from build123d import *

# Parameters (mm, degrees)
BOSS_EXTRUDE1_DEPTH = 2
EXTRUDE_1_DEPTH     = 5
EXTRUDE_2_DEPTH     = 5
SKETCH_4_R          = 14
SKETCH_4_R_2        = 14.00018903
CUT_EXTRUDE_1_DEPTH = 5
SKETCH1_3_R         = 10
CUT_EXTRUDE_2_DEPTH = 15
RIB_2_REACH         = 478.571
SKETCH_5_WALLS_W    = 5
SKETCH_5_WALLS_H    = 961.14191471
SKETCH_5_WALLS_H_2  = 961.14172568


with BuildPart() as part:
    # Sketch1 → Boss-Extrude1 (new, symmetric)
    with BuildSketch(Plane(origin=(0, 0, 0), x_dir=(0, 0, -1), z_dir=(1, 0, 0))):
        with BuildLine():
            Line((-48.878566689, 24.607830126), (451.121433311, 24.607830126))
            ThreePointArc((451.121433311, 24.607830126), (475.729263437, 0), (451.121433311, -24.607830126))
            Line((451.121433311, -24.607830126), (-48.878566689, -24.607830126))
            ThreePointArc((-48.878566689, -24.607830126), (-73.486396815, 0), (-48.878566689, 24.607830126))
        make_face()
    extrude(amount=BOSS_EXTRUDE1_DEPTH, both=True)

    # Sketch 1 → Extrude 1 (add)
    with BuildSketch(Plane(origin=(2, 0, 0), x_dir=(0, 0, -1), z_dir=(1, 0, 0))):
        with BuildLine():
            Line((451.121433311, 24.607830126), (-48.878566689, 24.607830126))
            ThreePointArc((-48.878566689, 24.607830126), (-73.486396815, 0), (-48.878566689, -24.607830126))
            Line((-48.878566689, -24.607830126), (451.121433311, -24.607830126))
            ThreePointArc((451.121433311, -24.607830126), (475.729263437, 0), (451.121433311, 24.607830126))
        make_face()
    extrude(amount=EXTRUDE_1_DEPTH)

    # Sketch 2 → Extrude 2 (add)
    with BuildSketch(Plane.ZY.offset(2)):
        with BuildLine():
            Line((-451.121433311, 24.607830126), (48.878566689, 24.607830126))
            ThreePointArc((48.878566689, 24.607830126), (73.486396815, 0), (48.878566689, -24.607830126))
            Line((48.878566689, -24.607830126), (-451.121433311, -24.607830126))
            ThreePointArc((-451.121433311, -24.607830126), (-475.729263437, 0), (-451.121433311, 24.607830126))
        make_face()
    extrude(amount=EXTRUDE_2_DEPTH)

    # Sketch 4 → Cut-Extrude 1 (cut)
    with BuildSketch(Plane.ZY.offset(7)):
        with BuildLine():
            ThreePointArc((48.878566689, 20), (68.878566689, 0), (48.878566689, -20))
            Line((48.878566689, -20), (-451.121433311, -20))
            ThreePointArc((-451.121433311, -20), (-471.121433311, 0), (-451.121433311, 20))
            Line((-451.121433311, 20), (48.878566689, 20))
        make_face()
        with Locations((48.878566689, 0)):
            Circle(SKETCH_4_R, mode=Mode.SUBTRACT)
        with Locations((-201.121433311, 0)):
            Circle(SKETCH_4_R_2, mode=Mode.SUBTRACT)
        with Locations((-451.121433311, 0)):
            Circle(SKETCH_4_R, mode=Mode.SUBTRACT)
    cut_extrude_1 = extrude(amount=-CUT_EXTRUDE_1_DEPTH, mode=Mode.SUBTRACT)

    # Mirror 1: Cut-Extrude 1 across plane
    add(cut_extrude_1.mirror(Plane.ZY), mode=Mode.SUBTRACT)

    # Sketch1_3 → Cut-Extrude 2 (cut, symmetric)
    with BuildSketch(Plane(origin=(0, 0, 0), x_dir=(0, 0, -1), z_dir=(1, 0, 0))):
        with Locations((-48.878566689, 0)):
            Circle(SKETCH1_3_R)
        with Locations((451.121433311, 0)):
            Circle(SKETCH1_3_R)
        with Locations((201.121433311, 0)):
            Circle(SKETCH1_3_R)
    extrude(amount=CUT_EXTRUDE_2_DEPTH, both=True, mode=Mode.SUBTRACT)

    # Sketch 5 walls → Rib 2 (add, up to next)
    with BuildSketch(Plane.ZY.offset(7), mode=Mode.PRIVATE) as rib_2_sk1:
        with Locations((48.878566689, 17)):
            Rectangle(SKETCH_5_WALLS_W, SKETCH_5_WALLS_H)
    rib_2_tool1 = extrude(rib_2_sk1.sketch, amount=-RIB_2_REACH, mode=Mode.PRIVATE) - part.part
    # Sketch 5 walls → Rib 2 (add, up to next)
    with BuildSketch(Plane.ZY.offset(7), mode=Mode.PRIVATE) as rib_2_sk2:
        with Locations((48.878566689, -17)):
            Rectangle(SKETCH_5_WALLS_W, SKETCH_5_WALLS_H)
    rib_2_tool2 = extrude(rib_2_sk2.sketch, amount=-RIB_2_REACH, mode=Mode.PRIVATE) - part.part
    # Sketch 5 walls → Rib 2 (add, up to next)
    with BuildSketch(Plane.ZY.offset(7), mode=Mode.PRIVATE) as rib_2_sk3:
        with Locations((-201.121433311, -17.000094515)):
            Rectangle(SKETCH_5_WALLS_W, SKETCH_5_WALLS_H_2)
    rib_2_tool3 = extrude(rib_2_sk3.sketch, amount=-RIB_2_REACH, mode=Mode.PRIVATE) - part.part
    # Sketch 5 walls → Rib 2 (add, up to next)
    with BuildSketch(Plane.ZY.offset(7), mode=Mode.PRIVATE) as rib_2_sk4:
        with Locations((-201.121433311, 17.000094515)):
            Rectangle(SKETCH_5_WALLS_W, SKETCH_5_WALLS_H_2)
    rib_2_tool4 = extrude(rib_2_sk4.sketch, amount=-RIB_2_REACH, mode=Mode.PRIVATE) - part.part
    # Sketch 5 walls → Rib 2 (add, up to next)
    with BuildSketch(Plane.ZY.offset(7), mode=Mode.PRIVATE) as rib_2_sk5:
        with Locations((-451.121433311, 17)):
            Rectangle(SKETCH_5_WALLS_W, SKETCH_5_WALLS_H)
    rib_2_tool5 = extrude(rib_2_sk5.sketch, amount=-RIB_2_REACH, mode=Mode.PRIVATE) - part.part
    # Sketch 5 walls → Rib 2 (add, up to next)
    with BuildSketch(Plane.ZY.offset(7), mode=Mode.PRIVATE) as rib_2_sk6:
        with Locations((-451.121433311, -17)):
            Rectangle(SKETCH_5_WALLS_W, SKETCH_5_WALLS_H)
    rib_2_tool6 = extrude(rib_2_sk6.sketch, amount=-RIB_2_REACH, mode=Mode.PRIVATE) - part.part
    rib_2_1 = rib_2_tool1.solids().sort_by_distance((-7, 17, 48.878566689))[0]
    add(rib_2_1)
    rib_2_2 = rib_2_tool2.solids().sort_by_distance((-7, -17, 48.878566689))[0]
    add(rib_2_2)
    rib_2_3 = rib_2_tool3.solids().sort_by_distance((-7, -17.000094515, -201.121433311))[0]
    add(rib_2_3)
    rib_2_4 = rib_2_tool4.solids().sort_by_distance((-7, 17.000094515, -201.121433311))[0]
    add(rib_2_4)
    rib_2_5 = rib_2_tool5.solids().sort_by_distance((-7, 17, -451.121433311))[0]
    add(rib_2_5)
    rib_2_6 = rib_2_tool6.solids().sort_by_distance((-7, -17, -451.121433311))[0]
    add(rib_2_6)
    rib_2 = rib_2_1 + rib_2_2 + rib_2_3 + rib_2_4 + rib_2_5 + rib_2_6  # Rib 2 as one shape, for the pattern or mirror that repeats it

    # Mirror 2: Rib 2 across plane
    add(rib_2.mirror(Plane.ZY))


solid = part.part
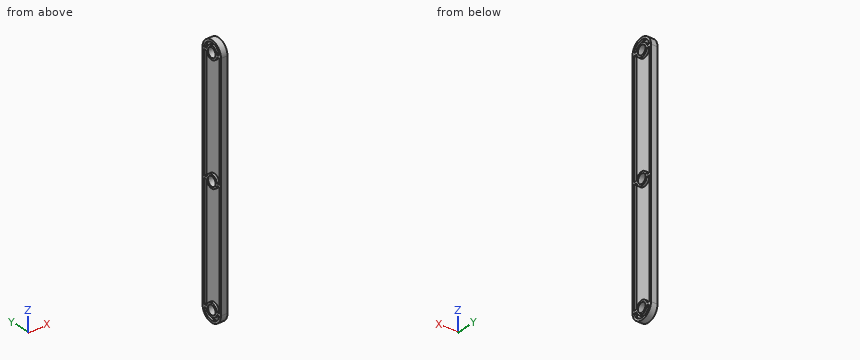
The model under review builds one solid part; all positions refer to its coordinate system, in mm. Round coordinates to 2 decimals unless told otherwise and drop trailing zeros. Loops run counter-clockwise (first coordinate to the right, second up) from the corner with the lowest first, then second, coordinate; pieces in that order, holes last. Notation, with made-up numbers: (2, 33.5) -> (43, 33.5) arc R6 ccw to (43, 42.5) -> close; hole circle Ø9 at (47.5, 10.5). An arc over 180 degrees is marked (long way). Return JSON: item names as keys, results as strings.
(1) For pin 1 (5 mm diameter, centred on x = -1, y = -16, fed in from -Z); pin 2 (2 mm diameter, centred on y = 3, z = -173, fed in from -X); pin 3 (1.5 mm diameter, centred on x = -4.5, y = -18, fed in from +Z), all flat-tipped, find the tip position at first contact; note any pin that passes through.
Solved:
{"pin 1": "z = -471.7", "pin 2": "x = -2", "pin 3": "z = 66.43"}
(2) Add section B-B on y = 0. State how many separate pieces and enclosed holes the cut face has, plus the area to 3 significant figures.
Solved:
{"separate pieces": "4", "enclosed holes": "0", "area": "2,290 mm2"}
(3) Add section A-A on z = -291. Write out the cut boundary in (x, y), plus the area to 3 significant figures.
Solved:
{"outline": "(-7, -24.61) -> (7, -24.61) -> (7, -20) -> (2, -20) -> (2, 20) -> (7, 20) -> (7, 24.61) -> (-7, 24.61) -> (-7, 20) -> (-2, 20) -> (-2, -20) -> (-7, -20) -> close", "area": "289 mm2"}
(4) For line 1 (Z direction, x = 1.5, y = 0.5); line 2 (Y direction, x = 3, z = -384.5); line 3 (Y direction, x = 5.75, z = -454), list the stretches that pass through material, from the lowest coordinate up.
Solved:
{"line 1": "-475.72 to -461.11, -441.13 to -211.11, -191.13 to 38.89, 58.87 to 73.48", "line 2": "-24.61 to -20, 20 to 24.61", "line 3": "-24.44 to -19.79, -13.7 to -9.58, 9.58 to 13.7, 19.79 to 24.44"}
